```python
from build123d import *

# Parameters (mm, degrees)
SKETCH1_R           = 50
SKETCH1_R_2         = 16.5
SKETCH1_R_3         = 1.55
SKETCH1_R_4         = 1.649528324
BOSS_EXTRUDE1_DEPTH = 10
SKETCH2_R           = 20
SKETCH2_R_2         = 16.1
BOSS_EXTRUDE2_DEPTH = 60
FILLET1_R           = 10


with BuildPart() as part:
    # Sketch1 → Boss-Extrude1 (new body)
    with BuildSketch(Plane.XY):
        Circle(SKETCH1_R)
        Circle(SKETCH1_R_2, mode=Mode.SUBTRACT)
        with Locations((-11.034036049, -39.098354169)):
            Circle(SKETCH1_R_3, mode=Mode.SUBTRACT)
        with Locations((-39.377185981, -9.99342156)):
            Circle(SKETCH1_R_4, mode=Mode.SUBTRACT)
        with Locations((-28.343149932, 29.104932609)):
            Circle(SKETCH1_R_3, mode=Mode.SUBTRACT)
        with Locations((11.034036049, 39.098354169)):
            Circle(SKETCH1_R_3, mode=Mode.SUBTRACT)
        with Locations((39.377185981, 9.99342156)):
            Circle(SKETCH1_R_3, mode=Mode.SUBTRACT)
        with Locations((28.343149932, -29.104932609)):
            Circle(SKETCH1_R_3, mode=Mode.SUBTRACT)
    extrude(amount=BOSS_EXTRUDE1_DEPTH)

    # Sketch2 → Boss-Extrude2 (add)
    with BuildSketch(Plane.XY.offset(10)):
        Circle(SKETCH2_R)
        Circle(SKETCH2_R_2, mode=Mode.SUBTRACT)
    extrude(amount=BOSS_EXTRUDE2_DEPTH)

    # Fillet1
    fillet1_edges = [part.edges().sort_by_distance(p)[0] for p in [
        (-20, 0, 10),
    ]]
    fillet(fillet1_edges, radius=FILLET1_R)


solid = part.part
```
Geometry check sheet. Reference: the model listing, model coordinates, mm. A direction names the side the tool comes from. Round coordinates to 2 decimals unless told otherwise and drop trailing zeros. Order: outer loops, then holes, each group sorted by start corner. A loop starts at its lowest first (then second) coordinate and runs counter-clockwise, first axis right, second up. Notation, with made-up numbers: (-29.75, -23.5) -> (4.25, -23.5) arc R19 cw to (4.25, -11.5) -> close; hole circle Ø11 at (-3, 56.25). An arc over 180 degrees is marked (long way). Return JSON: item names as keys, results as strings. Group by question number.
Q1. Section check D-D, the plane z = 15. Record the boundary of the cut face in (x, y).
Q2. Section check A-A, the plane y = 0. Record the boundary of the cut face in (x, z).
Q3. Section check C-C, the plane z = 35. Record the boundary of the cut face in (x, y), plus the area to 3 significant figures.
Q4. Tool access check on faces 5 (the cylindrical face through (-11.236, -37.562, 4.93)), 6 (the cylindrical face through (15.24, -6.32, 4.93)). Record the directions out of +Z, -Z, +X, -X, +Y, -Y that give a thin tool (end or side, any length) a straight path to the whole face; none if there is none.
Q5. Release check for a two-part mould opening along X. For faces 1 (the cylindrical face through (15.357, 4.836, 39.58)), 2 (the cylindrical face through (-4.336, -19.524, 44.65)), 3 (the flat face through (22, -22, 10)), 4 (the cylindrical face through (-37.804, -9.498, 4.93)) record: released by +X, released by -X, zero draft, split by the parting line, or undercut.
Q6. Material ranges on probe 1 along Y at (x, z) = (0, 34); probe 2 along Z at (x, y) = (19, 40); probe 3 along Y at (x, z) = (11, 6.5) (3 decimals), recorded low to high. Write a range as from..to.
Q7. Gauge pin test, flat ends, axial feed: pin 1 (4 mm diameter, centred on x = -28.34, y = 29.1, fed in from +Z); pin 2 (3 mm diameter, centred on x = -29.5, y = 4, fed in from +Z); pin 3 (5 mm diameter, centred on x = -23, z = 41.5, fed in from +Y); pin 4 (2 mm diameter, centred on x = 9.5, z = 58.5, fed in from +Y). Record the tip position at first contact, or that the pin passes through.
Numbers:
{
 "1": {"outline": "circle Ø42.68 at (0, 0); hole circle Ø32.2 at (0, 0)"},
 "2": {"outline": "(-50, 0) -> (-16.5, 0) -> (-16.5, 10) -> (-16.1, 10) -> (-16.1, 70) -> (-20, 70) -> (-20, 20) arc R10 cw to (-30, 10) -> (-50, 10) -> close; (16.1, 10) -> (16.5, 10) -> (16.5, 0) -> (50, 0) -> (50, 10) -> (30, 10) arc R10 cw to (20, 20) -> (20, 70) -> (16.1, 70) -> close"},
 "3": {"outline": "circle Ø40 at (0, 0); hole circle Ø32.2 at (0, 0)", "area": "442 mm^2"},
 "4": {"face 5": "+Z, -Z", "face 6": "-Z"},
 "5": {"face 1": "undercut", "face 2": "split by the parting line", "face 3": "zero draft", "face 4": "undercut"},
 "6": {"probe 1": "-20..-16.1, 16.1..20", "probe 2": "0..10", "probe 3": "-48.775..-12.298, 12.298..37.549, 40.648..48.775"},
 "7": {"pin 1": "z = 10", "pin 2": "z = 10.15", "pin 3": "through", "pin 4": "y = 18.1"}
}
